For this review, take the finished solid that the model builds, in its own axes (mm). A direction names the side the tool comes from. Round coordinates to 2 decimals unless told otherwise and drop trailing zeros. Loops run counter-clockwise (first coordinate to the right, second up) from the corner with the lowest first, then second, coordinate; pieces in that order, holes last.
1. Consider section A-A on z = 1.1. State the section outline as (x, y) points.
2. Consider section C-C on x = -2.35. State the section outline as (y, z) points.
3. Consider section D-D on x = -1.45. State the section outline as (y, z) points.
4. Draft analysis for pull direction Y (two halves, no side actions). For faces 3 (the cylindrical face through (0.044, 3.804, 0.493)), 4 (the flat face through (0, 0, 0)), 5 (the flat face through (0.6, 0, 1.2)), state which applies: released by +Y, released by -Y, zero draft, split by the parting line, or undercut.
5. To check wall thickness, follow line 1 along Y through (x, z) = (-0.9, 1.35); line 2 along X through (y, z) = (-2, 1.4); line 3 along Z through (x, y) = (-0.1, -0.75). State the ranges of each line that lie inside material, in increasing order.
6. Consider section B-B on y = 1.75. State the section outline as (x, z) points, then the cut area to 3 significant figures.
7. Tool access review of faces 1 (the flat face through (0, -3, 0.5)), 2 (the flat face through (-0.6, 0, 1.2)): name each direction out of +Z, -Z, +X, -X, +Y, -Y from which nothing blocks a thin tool from reaching the whole face with its end or side.
8. Clearance check with a flat-ended pin moving along its axis: pin 1 Ø1.8 at (x, y) = (0, 1) entering from +Z. State where the tip first meets the part, or that it passes through.
from build123d import *

# Parameters (mm, degrees)
PAD_DEPTH    = 1
PAD001_DEPTH = 0.5


with BuildPart() as part:
    # Sketch → Pad (new body)
    with BuildSketch(Plane.XY):
        with BuildLine():
            Line((3, 3), (3, -3))
            Line((3, -3), (-3, -3))
            Line((-3, -3), (-3, 3))
            ThreePointArc((3, 3), (0, 3.803848), (-3, 3))
        make_face()
    extrude(amount=PAD_DEPTH)

    # Sketch001 → Pad001 (new body)
    with BuildSketch(Plane.XY.offset(1)):
        Polygon((-2.5, 2.5), (-2.5, 1.5), (1.3, 1.5), (-2.5, -1.5), (-2.5, -2.5), (2.5, -2.5), (2.5, -1.5), (-1.3, -1.5), (2.5, 1.5), (2.5, 2.5), align=None)
    extrude(amount=PAD001_DEPTH)


solid = part.part
Resolved:
1. outline: (-2.5, -2.5) - (2.5, -2.5) - (2.5, -1.5) - (-1.3, -1.5) - (2.5, 1.5) - (2.5, 2.5) - (-2.5, 2.5) - (-2.5, 1.5) - (1.3, 1.5) - (-2.5, -1.5) - close
2. outline: (-3, 0) - (3.32, 0) - (3.32, 1) - (2.5, 1) - (2.5, 1.5) - (1.5, 1.5) - (1.5, 1) - (-1.38, 1) - (-1.38, 1.5) - (-2.5, 1.5) - (-2.5, 1) - (-3, 1) - close
3. outline: (-3, 0) - (3.63, 0) - (3.63, 1) - (2.5, 1) - (2.5, 1.5) - (1.5, 1.5) - (1.5, 1) - (-0.67, 1) - (-0.67, 1.5) - (-2.5, 1.5) - (-2.5, 1) - (-3, 1) - close
4. face 3: released by +Y
4. face 4: zero draft
4. face 5: undercut
5. line 1: y = -2.5 to -1.5, -1.18 to -0.24, 1.5 to 2.5
5. line 2: x = -2.5 to 2.5
5. line 3: z = 0 to 1
6. outline: (-3, 0) - (3, 0) - (3, 1) - (2.5, 1) - (2.5, 1.5) - (-2.5, 1.5) - (-2.5, 1) - (-3, 1) - close
6. area: 8.50 mm2
7. face 1: +Z, -Z, +X, -X, -Y
7. face 2: +Z, -X
8. pin 1: stops at z = 1.5
